```python
from build123d import *

# Parameters (mm, degrees)
ESQUISSE1_R        = 5.5
BOSS_EXTRU_1_DEPTH = 5
ESQUISSE2_W        = 10
ESQUISSE2_H        = 38
ESQUISSE2_W_2      = 38
ESQUISSE2_H_2      = 10
BOSS_EXTRU_2_DEPTH = 6
D_POUILLE3_ANGLE   = 10
BOSS_EXTRU_3_DEPTH = 10
CHANFREIN1_SIZE    = 5


with BuildPart() as part:
    # Esquisse1 → Boss.-Extru.1 (new body)
    with BuildSketch(Plane.XY):
        Polygon((0, 0), (0, 90), (45, 90), (135, 45), (135, 0), align=None)
        with Locations((22.5, 75)):
            Circle(ESQUISSE1_R, mode=Mode.SUBTRACT)
        with Locations((22.5, 15)):
            Circle(ESQUISSE1_R, mode=Mode.SUBTRACT)
        with Locations((120, 22.5)):
            Circle(ESQUISSE1_R, mode=Mode.SUBTRACT)
        with Locations((60, 22.5)):
            Circle(ESQUISSE1_R, mode=Mode.SUBTRACT)
    extrude(amount=BOSS_EXTRU_1_DEPTH)

    # Esquisse2 → Boss.-Extru.2 (add)
    with BuildSketch(Plane.XY.offset(5)):
        with Locations((22.5, 45)):
            Rectangle(ESQUISSE2_W, ESQUISSE2_H)
        with Locations((90, 22.5)):
            Rectangle(ESQUISSE2_W_2, ESQUISSE2_H_2)
    extrude(amount=BOSS_EXTRU_2_DEPTH)

    # Dépouille3
    d_pouille3_faces = [part.faces().sort_by_distance(p)[0] for p in [
        (90, 27.5, 8),
        (109, 22.5, 8),
        (71, 22.5, 8),
        (90, 17.5, 8),
        (22.5, 26, 8),
        (27.5, 45, 8),
        (22.5, 64, 8),
        (17.5, 45, 8),
    ]]
    draft(d_pouille3_faces, Plane.XY.offset(5), D_POUILLE3_ANGLE)

    # Esquisse3 → Boss.-Extru.3 (add)
    with BuildSketch(Plane.XY.offset(5)):
        Polygon((45, 90), (45, 45), (135, 45), align=None)
    extrude(amount=BOSS_EXTRU_3_DEPTH)

    # Chanfrein1
    chanfrein1_edges = [part.edges().sort_by_distance(p)[0] for p in [
        (45, 45, 10),
    ]]
    chamfer(chanfrein1_edges, length=CHANFREIN1_SIZE)


solid = part.part
```
Can you work these out from the model? Positions are in its coordinate system, mm. A direction names the side the tool comes from. Coordinates: 2 decimals unless noted, no trailing zeros. Write each loop counter-clockwise with the first axis right and the second up, starting at its lowest first coordinate (ties: lowest second). Pieces come first, ordered by that corner, then holes. Notation, with made-up numbers: M -38,49 L -29,49 A22 cw -29,61 Z; hole C 61.25,17.25 d3. An arc over 180 degrees is marked long. Write item = value, one per line. Start each with the question number.
Q1. If I drill on L1, parallel to Y at x = 22.5, z = 1.55; L2, parallel to Z at x = 15, y = 42.5; L3, parallel to Y at x = 60, z = 2.9, over which ranges is the centre line in solid material (lowest first)? Write a range as [from, to].
Q2. If we section it at C-C, the plane y = 22.5: Write out the boundary of the cut face in (x, z).
Q3. I'm going to push flat-ended pins straight in: pin 1 (6 mm diameter, centred on x = 34, y = 68, fed in from -Z); pin 2 (4 mm diameter, centred on x = 94, y = 22.5, fed in from +Z); pin 3 (6.5 mm diameter, centred on x = 60, y = 22.5, fed in from +Z); pin 4 (6 mm diameter, centred on y = 55.5, z = 7.5, fed in from +X). Where does each tip first touch, or does it pass through?
Q4. Thinking about a two-plate mould opening in Y: for faces 1 (the face through (22.43, 26.52, 7.96)), 2 (the face through (21.784, 80.453, 2.465)), 3 (the face through (18.02, 44.73, 7.96)), 4 (the face through (54.505, 22.742, 2.465)), which applies, released by +Y, released by -Y, zero draft, split by the parting line, or undercut?
Q5. If we section it at B-B, the plane z = 2.75: Write out the boundary of the cut face in (x, y).
Q6. If we section it at D-D, the plane x = 22.5: Write out the boundary of the cut face in (y, z), then the cut area to 3 significant figures.
Q7. If we section it at A-A, the plane x = 120: Write out the boundary of the cut face in (y, z).
Q8. On a 3-axis mill with a long thin cutter (end or side, diameter ignored), from which of +Z, -Z, +X, -X, +Y, -Y can I reach the whole of each face in a straight line? I mean faces 5 (the face through (22, 45, 11)), 6 (the face through (26.98, 44.73, 7.96)), 7 (the face through (48, 47, 10)), 8 (the face through (92, 45, 10)). Say none if no direction works.
Check sheet entries:
q1.L1 = [0, 9.5], [20.5, 69.5], [80.5, 90]
q1.L2 = [0, 5]
q1.L3 = [0, 17], [28, 82.5]
q2.outline = M 0,0 L 54.5,0 L 54.5,5 L 0,5 Z; M 65.5,0 L 114.5,0 L 114.5,5 L 109,5 L 107.94,11 L 72.06,11 L 71,5 L 65.5,5 Z; M 125.5,0 L 135,0 L 135,5 L 125.5,5 Z
q3.pin_1 = 0
q3.pin_2 = 11
q3.pin_3 = through
q3.pin_4 = 120
q4.face_1 = released by -Y
q4.face_2 = undercut
q4.face_3 = zero draft
q4.face_4 = undercut
q5.outline = M 0,0 L 135,0 L 135,45 L 45,90 L 0,90 Z; hole C 22.5,15 d11; hole C 22.5,75 d11; hole C 60,22.5 d11; hole C 120,22.5 d11
q6.outline = M 0,0 L 9.5,0 L 9.5,5 L 0,5 Z; M 20.5,0 L 69.5,0 L 69.5,5 L 64,5 L 62.94,11 L 27.06,11 L 26,5 L 20.5,5 Z; M 80.5,0 L 90,0 L 90,5 L 80.5,5 Z
q6.area = 562 mm²
q7.outline = M 0,0 L 17,0 L 17,5 L 0,5 Z; M 28,0 L 52.5,0 L 52.5,15 L 45,15 L 45,5 L 28,5 Z
q8.face_5 = +Z, -X, +Y, -Y
q8.face_6 = +Z, +Y, -Y
q8.face_7 = +Z, -Y
q8.face_8 = +Z, +X
